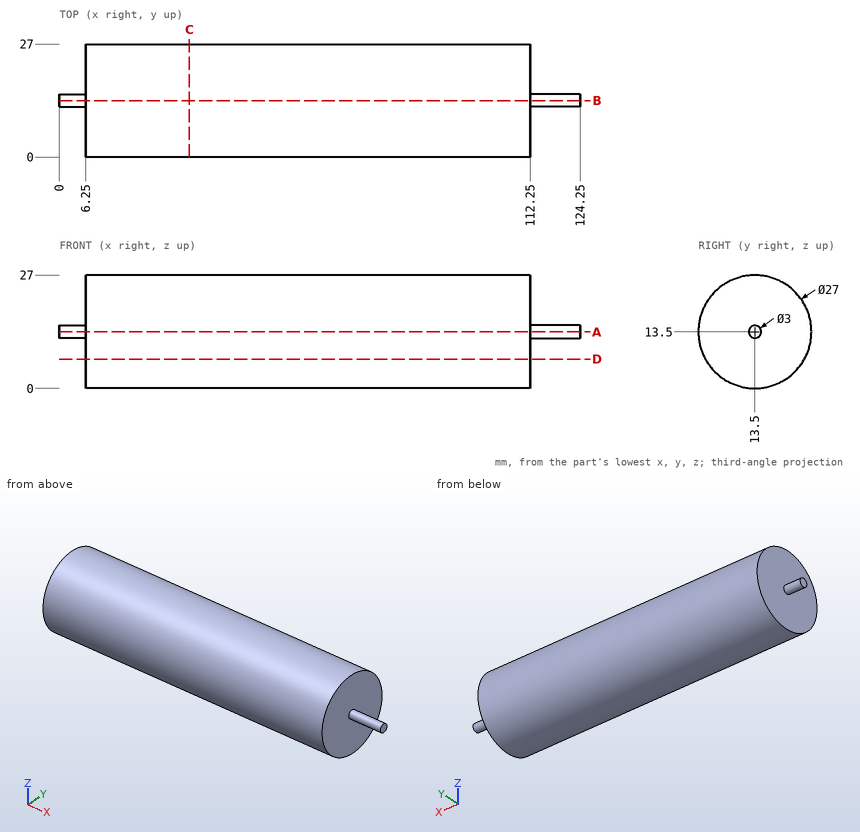
Input: dimensioned drawing with shaded views. Units: mm. Origin: part minimum x, y, z. Coordinates: 2 decimals unless noted, no trailing zeros. Loops run counter-clockwise (first coordinate to the right, second up) from the corner with the lowest first, then second, coordinate; pieces in that order, holes last. Notation, with made-up numbers: M 83,17.25 L 91,17.25 A28 ccw 91,47.25 Z; hole C -35.5,12.5 d7. An arc over 180 degrees is marked long. Put each result on its own line as item: value.
(1) First-contact query: pin 1 (1.5 mm diameter, centred on y = 10, z = 11.5, fed in from +X); pin 2 (2 mm diameter, centred on x = 18, y = 8, fed in from +Z); pin 3 (10 mm diameter, centred on x = 110, y = 5.5, fed in from -Z); pin 4 (5 mm diameter, centred on x = 13, z = 11, fed in from -Y). Flat tips, straight axial feed; report the tip coordinate or a pass-through.
Answer sheet:
pin 1: stops at x = 112.25
pin 2: stops at z = 26.23
pin 3: stops at z = 0.34
pin 4: stops at y = 0
(2) Cut plane D-D on z = 7. Return the cut outline in (x, y), then the cut area to 3 significant figures.
Answer sheet:
outline: M 6.25,1.67 L 112.25,1.67 L 112.25,25.33 L 6.25,25.33 Z
area: 2,510 mm^2
(3) Cut plane A-A on z = 13.5. Return the cut outline in (x, y), then the cut area to 3 significant figures.
Answer sheet:
outline: M 0,12 L 6.25,12 L 6.25,0 L 112.25,0 L 112.25,12 L 124.25,12 L 124.25,15 L 112.25,15 L 112.25,27 L 6.25,27 L 6.25,15 L 0,15 Z
area: 2,920 mm^2
(4) Cut plane C-C on x = 31. Return the cut outline in (y, z).
Answer sheet:
outline: C 13.5,13.5 d27
(5) Material intervals for probe 1 along X at (y, z) = (17, 23); probe 2 along Z at (x, y) = (102, 13.75); probe 3 along Y at (x, z) = (23, 8.75), sorted ascending.
Answer sheet:
probe 1: x = 6.25 to 112.25
probe 2: z = 0 to 27
probe 3: y = 0.86 to 26.14
